from build123d import *

# Parameters (mm, degrees)
CROQUIS1_R              = 5.6
CROQUIS1_R_2            = 7.5
SALIENTE_EXTRUIR1_DEPTH = 54
CROQUIS6_W              = 54
CROQUIS6_H              = 70
SALIENTE_EXTRUIR3_DEPTH = 74
CORTAR_EXTRUIR13_DEPTH  = 74
CORTAR_EXTRUIR14_DEPTH  = 74
CROQUIS9_W              = 3
CROQUIS9_H              = 11.2
CORTAR_EXTRUIR15_DEPTH  = 74
CROQUIS10_R             = 5.6
CORTAR_EXTRUIR16_DEPTH  = 74
CROQUIS11_R             = 10
CROQUIS11_R_2           = 5.6
SALIENTE_EXTRUIR4_DEPTH = 5
CROQUIS12_R             = 10
CROQUIS12_R_2           = 5.6
SALIENTE_EXTRUIR5_DEPTH = 5
CROQUIS13_W             = 50
CROQUIS13_H             = 73
CORTAR_EXTRUIR17_DEPTH  = 74
CROQUIS14_W             = 74
CROQUIS14_H             = 73
SALIENTE_EXTRUIR6_DEPTH = 54
CORTAR_EXTRUIR18_DEPTH  = 54
REDONDEO3_R             = 2
REDONDEO4_R             = 2


with BuildPart() as part:
    # Croquis1 → Saliente-Extruir1 (new body)
    with BuildSketch(Plane.XY):
        with BuildLine():
            Line((0, 143), (0, 70))
            add(Edge.make_bspline(
                [(22, 15), (22, 22.317960933), (17.777719643, 44.524463784), (15.903513438, 66.300635574), (0, 70)],
                knots=[0, 0, 0, 0, 0.399675276, 1, 1, 1, 1], degree=3))
            ThreePointArc((22, 15), (37, 0), (52, 15))
            add(Edge.make_bspline(
                [(52, 15), (52, 22.317960933), (56.222280357, 44.524463784), (58.096486562, 66.300635574), (74, 70)],
                knots=[0, 0, 0, 0, 0.399675276, 1, 1, 1, 1], degree=3))
            Line((74, 70), (74, 143))
            ThreePointArc((74, 143), (37, 180), (0, 143))
        make_face()
        with Locations((37, 15)):
            Circle(CROQUIS1_R, mode=Mode.SUBTRACT)
        with Locations((37, 155)):
            Circle(CROQUIS1_R_2, mode=Mode.SUBTRACT)
    extrude(amount=SALIENTE_EXTRUIR1_DEPTH)

    # Croquis6 → Saliente-Extruir3 (add)
    with BuildSketch(Plane.ZY):
        with Locations((27, 35)):
            Rectangle(CROQUIS6_W, CROQUIS6_H)
    extrude(amount=-SALIENTE_EXTRUIR3_DEPTH)

    # Croquis7 → Cortar-Extruir13 (cut)
    with BuildSketch(Plane(origin=(74, 0, 0), x_dir=(0, 0, -1), z_dir=(1, 0, 0))):
        Polygon((-52, 0), (-2, 0), (-2, 9.4), (-5, 9.4), (-5, 20.6), (-2, 20.6), (-2, 70), (-52, 70), (-52, 20.6), (-49, 20.6), (-49, 9.4), (-52, 9.4), align=None)
    extrude(amount=-CORTAR_EXTRUIR13_DEPTH, mode=Mode.SUBTRACT)

    # Croquis8 → Cortar-Extruir14 (cut)
    with BuildSketch(Plane(origin=(0, 0, 0), x_dir=(-1, 0, 0), z_dir=(0, 0, -1))):
        with BuildLine():
            add(Edge.make_bspline(
                [(-74, 70), (-58.096486562, 66.300635574), (-56.222280357, 44.524463784), (-52, 22.317960933), (-52, 15)],
                knots=[0, 0, 0, 0, 0.600324724, 1, 1, 1, 1], degree=3))
            Line((-74, 70), (-74, 0))
            Line((-74, 0), (-37, 0))
            ThreePointArc((-37, 0), (-47.606601718, 4.393398282), (-52, 15))
        make_face()
        with BuildLine():
            ThreePointArc((-22, 15), (-26.393398282, 4.393398282), (-37, 0))
            Line((-37, 0), (0, 0))
            Line((0, 0), (0, 70))
            add(Edge.make_bspline(
                [(-22, 15), (-22, 22.317960933), (-17.777719643, 44.524463784), (-15.903513438, 66.300635574), (0, 70)],
                knots=[0, 0, 0, 0, 0.399675276, 1, 1, 1, 1], degree=3))
        make_face()
    extrude(amount=-CORTAR_EXTRUIR14_DEPTH, mode=Mode.SUBTRACT)

    # Croquis9 → Cortar-Extruir15 (cut)
    with BuildSketch(Plane(origin=(74, 0, 0), x_dir=(0, 0, -1), z_dir=(1, 0, 0))):
        with Locations((-50.5, 15)):
            Rectangle(CROQUIS9_W, CROQUIS9_H)
        Polygon((-2, 20.6), (-5.198845147, 20.6), (-5, 9.4), (-2, 9.4), align=None)
    extrude(amount=-CORTAR_EXTRUIR15_DEPTH, mode=Mode.SUBTRACT)

    # Croquis10 → Cortar-Extruir16 (cut)
    with BuildSketch(Plane(origin=(0, 0, 0), x_dir=(-1, 0, 0), z_dir=(0, 0, -1))):
        with Locations((-37, 15)):
            Circle(CROQUIS10_R)
    extrude(amount=-CORTAR_EXTRUIR16_DEPTH, mode=Mode.SUBTRACT)

    # Croquis11 → Saliente-Extruir4 (add)
    with BuildSketch(Plane(origin=(0, 0, 52), x_dir=(-1, 0, 0), z_dir=(0, 0, -1))):
        with Locations(Location((-37, 15, 0), (0, 0, 270))):
            Circle(CROQUIS11_R)
        with Locations((-37, 15)):
            Circle(CROQUIS11_R_2, mode=Mode.SUBTRACT)
    extrude(amount=SALIENTE_EXTRUIR4_DEPTH)

    # Croquis12 → Saliente-Extruir5 (add)
    with BuildSketch(Plane.XY.offset(2)):
        with Locations(Location((37, 15, 0), (0, 0, 270))):
            Circle(CROQUIS12_R)
        with Locations(Location((37, 15, 0), (0, 0, 180))):
            Circle(CROQUIS12_R_2, mode=Mode.SUBTRACT)
    extrude(amount=SALIENTE_EXTRUIR5_DEPTH)

    # Croquis13 → Cortar-Extruir17 (cut)
    with BuildSketch(Plane.ZY):
        with Locations((27, 106.5)):
            Rectangle(CROQUIS13_W, CROQUIS13_H)
    extrude(amount=-CORTAR_EXTRUIR17_DEPTH, mode=Mode.SUBTRACT)

    # Croquis14 → Saliente-Extruir6 (add)
    with BuildSketch(Plane(origin=(0, 0, 0), x_dir=(-1, 0, 0), z_dir=(0, 0, -1))):
        with Locations((-37, 106.5)):
            Rectangle(CROQUIS14_W, CROQUIS14_H)
    extrude(amount=-SALIENTE_EXTRUIR6_DEPTH)

    # Croquis15 → Cortar-Extruir18 (cut)
    with BuildSketch(Plane.XY.offset(54)):
        with BuildLine():
            Line((9.470720421, 142.990900166), (9.470720421, 62.137684014))
            Line((9.470720421, 62.137684014), (-11.518865127, 62.137684014))
            Line((-11.518865127, 62.137684014), (-11.518865127, 188.692436646))
            Line((-11.518865127, 188.692436646), (98.86488905, 188.692436646))
            Line((98.86488905, 188.692436646), (98.86488905, 62.137684014))
            Line((98.86488905, 62.137684014), (64.470720421, 62.137684014))
            Line((64.470720421, 62.137684014), (64.470720421, 142.990900166))
            ThreePointArc((64.470720421, 142.990900166), (36.970720421, 170.490900166), (9.470720421, 142.990900166))
        make_face()
    extrude(amount=-CORTAR_EXTRUIR18_DEPTH, mode=Mode.SUBTRACT)

    # Redondeo3
    redondeo3_edges = [part.edges().sort_by_distance(p)[0] for p in [
        (9.470720421, 104.272545077, 54),
        (36.970720421, 170.490900166, 54),
        (64.470720421, 104.24810361, 54),
    ]]
    fillet(redondeo3_edges, radius=REDONDEO3_R)

    # Redondeo4
    redondeo4_edges = [part.edges().sort_by_distance(p)[0] for p in [
        (36.970720421, 170.490900166, 0),
        (9.470720421, 104.272545072, 0),
        (64.470720421, 104.248103603, 0),
    ]]
    fillet(redondeo4_edges, radius=REDONDEO4_R)


solid = part.part
Could you check a few things on this model? Use its own coordinates, in mm. A direction names the side the tool comes from. Give positions to 0.01 mm unless a question says otherwise; leave off trailing zeros. Order: outer loops, then holes, each group sorted by start corner. A loop starts at its lowest first (then second) coordinate and runs counter-clockwise, first axis right, second up. Notation, with made-up numbers: (55.5, 25) -> (112.5, 25) arc R31 ccw to (112.5, 59) -> close; hole circle Ø3 at (16.5, 27). An arc over 180 degrees is marked (long way). Answer in a Markdown table with one row per item. Add a question column.
Item 1: For faces 1 (the flat face through (9.471, 107, 27)), 2 (the flat face through (41.3, 10.7, 47)), 3 (the cylindrical face through (45.872, 10.386, 49.535)), which set-ups out of +Z, -Z, +X, -X, +Y, -Y let a thin tool reach every point of the face, with its end or its side?
Item 2: We'd pull the mould along Z, two halves only. Please class faces 4 (the flat face through (37, 70, 27)), 5 (the cylindrical face through (28.128, 10.386, 4.465)), 6 (the flat face through (37, 83, 54)), 7 (the cylindrical face through (36.024, 162.436, 26.622)): pulls with the +Z half, pulls with the -Z half, needs draft (parallel to the pull), parting line crosses it, or undercut.
Item 3: Please list where these lines run through material, in increasing order: probe 1 along Y at (x, z) = (37, 49.65); probe 2 along Y at (x, z) = (37, 53); probe 3 along Z at (x, y) = (48, 64.5).
Item 4: Imagine slicing it at B-B (z = 11). List the corners of the cut face in (x, y) for me.
Item 5: Imagine slicing it at A-A (y = 68). List the corners of the cut face in (x, z) for me, and give its area (3 significant figures).
Item 6: I'm going to push flat-ended pins straight in: P1, Ø3, axis at x = 18, z = 23.5, coming from the +Y side; P2, Ø1, axis at x = 22, z = 24.5, coming from the -Y side; P3, Ø2, axis at x = 23.5, z = 37, coming from the +Y side. Where does each tip first touch, or does it pass through?
Item 7: Imagine slicing it at C-C (y = 17). Count the separate pieces of the cut face and the enclosed holes in it, and give its area (3 significant figures).
Result:
| question | item | result |
|---|---|---|
| 1 | face 1 | +Z, -Z, -X, +Y, -Y |
| 1 | face 2 | +X, -X, -Y |
| 1 | face 3 | none |
| 2 | face 4 | undercut |
| 2 | face 5 | undercut |
| 2 | face 6 | pulls with the +Z half |
| 2 | face 7 | needs draft |
| 3 | probe 1 | 5 to 9.4, 20.6 to 25, 70 to 147.5, 162.5 to 170.49 |
| 3 | probe 2 | 0 to 9.4, 20.6 to 147.5, 162.5 to 170.22 |
| 3 | probe 3 | 0 to 2, 52 to 54 |
| 4 | outline | (9.47, 70) -> (64.47, 70) -> (64.47, 142.99) arc R27.5 ccw to (9.47, 142.99) -> close; hole circle Ø15 at (37, 155) |
| 5 | outline | (9.47, 2) arc R2 ccw to (11.47, 0) -> (62.47, 0) arc R2 ccw to (64.47, 2) -> close; (9.47, 52) -> (64.47, 52) arc R2 ccw to (62.47, 54) -> (11.47, 54) arc R2 ccw to start |
| 5 | area | 217 mm2 |
| 6 | P1 | y = 164.23 |
| 6 | P2 | y = 70 |
| 6 | P3 | y = 167.5 |
| 7 | separate pieces | 4 |
| 7 | enclosed holes | 0 |
| 7 | area | 170 mm2 |
